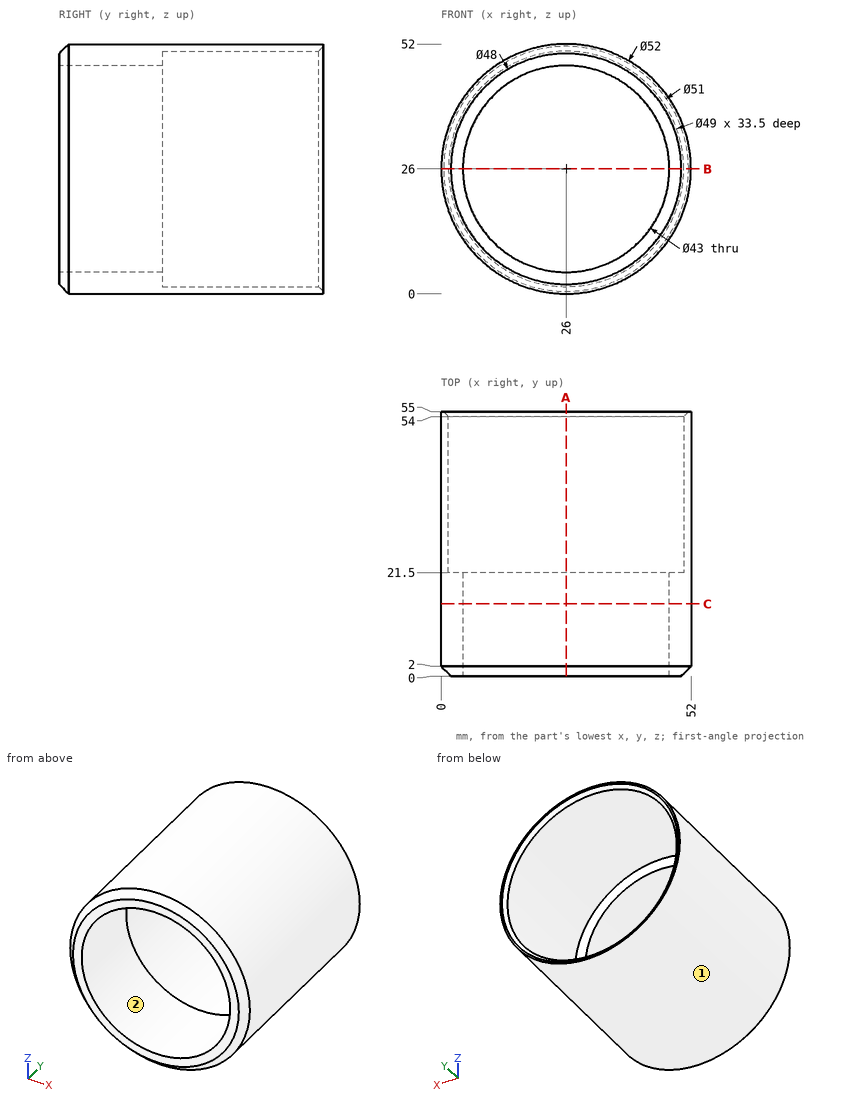
Drawing for the job (mm, zero at the part's lowest x, y, z). Give positions to 0.01 mm unless a question says otherwise; leave off trailing zeros. Write each loop counter-clockwise with the first axis right and the second up, starting at its lowest first coordinate (ties: lowest second). Pieces come first, ordered by that corner, then holes. Notation, with made-up numbers: (-40, 7.5) - (-13, 7.5) arc R32 cw to (-13, 36.5) - close; hole circle Ø1 at (3, 7). An arc over 180 degrees is marked (long way). Answer as CSV lines item,"result".
Q1. Pull direction X, two halves, no side cores. Call the marked faces 1 and 2: released by +X, released by -X, zero draft, split by the parting line, or undercut.
Result set:
face 1,"split by the parting line"
face 2,"undercut"
Q2. Drill centre lines: line 1 (Z direction, x = 26, y = 46); line 2 (Z direction, x = 21, y = 22.5); line 3 (Y direction, x = 10.5, z = 9). Where is each one in solid material? Low to high. Write a range as from..to.
Result set:
line 1,"0..1.5, 50.5..52"
line 2,"0.49..2.02, 49.98..51.51"
line 3,"0..21.5"
Q3. Band-saw the part on A-A (x = 26). Give the cut face in (y, z).
Result set:
outline,"(0, 2) - (2, 0) - (55, 0) - (55, 0.5) - (54, 1.5) - (21.5, 1.5) - (21.5, 4.5) - (0, 4.5) - close; (0, 47.5) - (21.5, 47.5) - (21.5, 50.5) - (54, 50.5) - (55, 51.5) - (55, 52) - (2, 52) - (0, 50) - close"
Q4. Band-saw the part on C-C (y = 15). Give the cut face in (x, z), and give its area (3 significant figures).
Result set:
outline,"circle Ø52 at (26, 26); hole circle Ø43 at (26, 26)"
area,"672 mm²"
Q5. Band-saw the part on B-B (z = 26). Give the cut face in (x, y), and give its area (3 significant figures).
Result set:
outline,"(0, 2) - (2, 0) - (4.5, 0) - (4.5, 21.5) - (1.5, 21.5) - (1.5, 54) - (0.5, 55) - (0, 55) - close; (47.5, 0) - (50, 0) - (52, 2) - (52, 55) - (51.5, 55) - (50.5, 54) - (50.5, 21.5) - (47.5, 21.5) - close"
area,"289 mm²"
Q6. Flat gauge pins, fed straight in: pin 1 Ø1.5 at (y, z) = (26.5, 35.5) entering from -X; pin 2 Ø1 at (x, y) = (11.5, 15.5) entering from +Z; pin 3 Ø3 at (x, y) = (22, 28) entering from +Z. Where does each tip first touch, or does it go through?
Result set:
pin 1,"x = 1.52"
pin 2,"z = 47.91"
pin 3,"z = 51.88"
